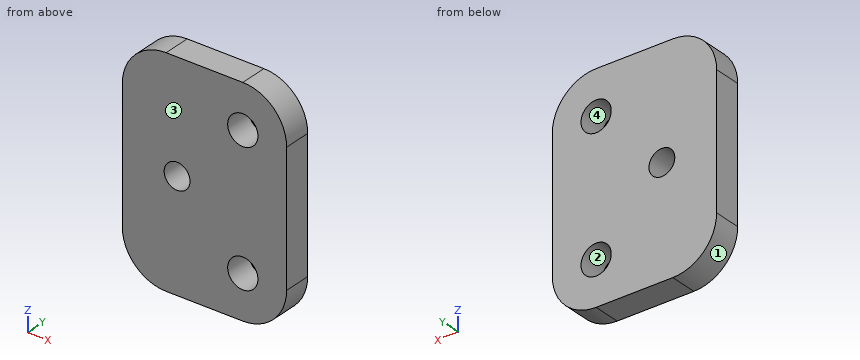
from build123d import *

# Parameters (mm, degrees)
F0_W     = 19.05
F0_H     = 25.4
F0_R     = 1.5
F0_R_2   = 1.7526
F1_DEPTH = 3.175
F2_R     = 5.08


with BuildPart() as f1:
    # F0 (on Front) → F1 (new body)
    with BuildSketch(Plane.XZ):
        with Locations((3.175, 0)):
            Rectangle(F0_W, F0_H)
        Circle(F0_R, mode=Mode.SUBTRACT)
        with Locations((7.62, -7.62)):
            Circle(F0_R_2, mode=Mode.SUBTRACT)
        with Locations((7.62, 7.62)):
            Circle(F0_R_2, mode=Mode.SUBTRACT)
    extrude(amount=F1_DEPTH)

    # F2
    f2_edges = [f1.edges().sort_by_distance(p)[0] for p in [
        (12.7, -1.5875, 12.7),
        (12.7, -1.5875, -12.7),
        (-6.35, -1.5875, 12.7),
        (-6.35, -1.5875, -12.7),
    ]]
    fillet(f2_edges, radius=F2_R)


solid = f1.part
The listing builds one solid part. Answer for the finished solid, in the listing's coordinates (mm). Face numbers are marked on the shaded views. Give positions to 0.01 mm unless a question says otherwise; leave off trailing zeros. Write each loop counter-clockwise with the first axis right and the second up, starting at its lowest first coordinate (ties: lowest second). Pieces come first, ordered by that corner, then holes. Notation, with made-up numbers: (69, -27) -> (116, -27) arc R21 cw to (116, -14) -> close; hole circle Ø7 at (20.5, -35). An arc over 180 degrees is marked (long way). Use a Markdown table: item, result.
(1) Section D-D, the plane z = -10.75 is taken. Determine the outline of the cut face in (x, y) (3 decimals).
Return value:
| item | result |
|---|---|
| outline | (-5.271, -3.175) -> (11.621, -3.175) -> (11.621, 0) -> (-5.271, 0) -> close |
(2) Section B-B, the plane z = 0 is taken. Determine the outline of the cut face in (x, y) (3 decimals).
Return value:
| item | result |
|---|---|
| outline | (-6.35, -3.175) -> (-1.5, -3.175) -> (-1.5, 0) -> (-6.35, 0) -> close; (1.5, -3.175) -> (12.7, -3.175) -> (12.7, 0) -> (1.5, 0) -> close |
(3) Section A-A, the plane x = 0 is taken. Determine the outline of the cut face in (y, z) (3 decimals), then the cut area to 3 significant figures.
Return value:
| item | result |
|---|---|
| outline | (-3.175, -12.7) -> (0, -12.7) -> (0, -1.5) -> (-3.175, -1.5) -> close; (-3.175, 1.5) -> (0, 1.5) -> (0, 12.7) -> (-3.175, 12.7) -> close |
| area | 71.1 mm2 |
(4) Find the intervals of material crossed by probe 1 along X at (y, z) = (-0.2, 7.75); probe 2 along X at (y, z) = (-2.35, 10.75); probe 3 along Z at (x, y) = (-0.25, -0.3), in increasing order. Write a range as from..to.
Return value:
| item | result |
|---|---|
| probe 1 | -6.35..5.87, 9.37..12.7 |
| probe 2 | -5.27..11.62 |
| probe 3 | -12.7..-1.48, 1.48..12.7 |
(5) Section C-C, the plane y = -2.05 is taken. Determine the outline of the cut face in (x, z), then the cut area to 3 significant figures.
Return value:
| item | result |
|---|---|
| outline | (-6.35, -7.62) arc R5.08 ccw to (-1.27, -12.7) -> (7.62, -12.7) arc R5.08 ccw to (12.7, -7.62) -> (12.7, 7.62) arc R5.08 ccw to (7.62, 12.7) -> (-1.27, 12.7) arc R5.08 ccw to (-6.35, 7.62) -> close; hole circle Ø3 at (0, 0); hole circle Ø3.51 at (7.62, -7.62); hole circle Ø3.51 at (7.62, 7.62) |
| area | 435 mm2 |
(6) Determine the mould class of the marked faces 1, 2, 3 and 4 for opening direction Z: released by +Z, released by -Z, zero draft, split by the parting line, or undercut.
Return value:
| item | result |
|---|---|
| face 1 | released by -Z |
| face 2 | undercut |
| face 3 | zero draft |
| face 4 | undercut |
